Here's how the part is built. I have some questions about the finished solid (model axes, mm). Face numbers are marked on the shaded views. A direction names the side the tool comes from. Round coordinates to 2 decimals unless told otherwise and drop trailing zeros. Write each loop counter-clockwise with the first axis right and the second up, starting at its lowest first coordinate (ties: lowest second). Pieces come first, ordered by that corner, then holes. Notation, with made-up numbers: M 2.25,-23 L 17.25,-23 A9 ccw 17.25,-16 Z; hole C 28,72 d8. An arc over 180 degrees is marked long. Use a Markdown table: item, result. Add a question column.
Autodesk Inventor part; units mm, degrees
ref_plane "YZ Plane" through (0, 0, 0) normal (1, 0, 0) x (0, 1, 0)
ref_plane "XZ Plane" through (0, 0, 0) normal (0, 1, 0) x (-1, 0, 0)
ref_plane "XY Plane" through (0, 0, 0) normal (0, 0, 1) x (1, 0, 0)
sketch "Boceto1" plane through (0, 0, 0) normal (0, 1, 0) x (-1, 0, 0)
  line L0 (0, 0) -> (-200, 0)
  line L1 (-200, 0) -> (-200, -140)
  line L2 (-200, -140) -> (0, -140)
  line L3 (0, -140) -> (0, 0)
  line L4 (0, 0) -> (-200, 0)
  line L5 (-200, 0) -> (-200, -10)
  line L6 (-200, -10) -> (0, -10)
  line L7 (0, -10) -> (0, 0)
  line L8 (0, -140) -> (-200, -140)
  line L9 (-200, -140) -> (-200, -130)
  line L10 (-200, -130) -> (0, -130)
  line L11 (0, -130) -> (0, -140)
  dimension "d0" = 200
  dimension "d1" = 140
  dimension "d2" = 200
  dimension "d3" = 10
  dimension "d4" = 200
  dimension "d5" = 10
extrude "Extrusión1" add sketch "Boceto1" along normal blind 10 contours L3 L10 L1 L6
extrude "Extrusión2" add sketch "Boceto1" along normal blind 70 contours L3 L6 L1 L0 | L3 L2 L1 L10
properties part number "Soporte_rods" material "Acero, fundido"
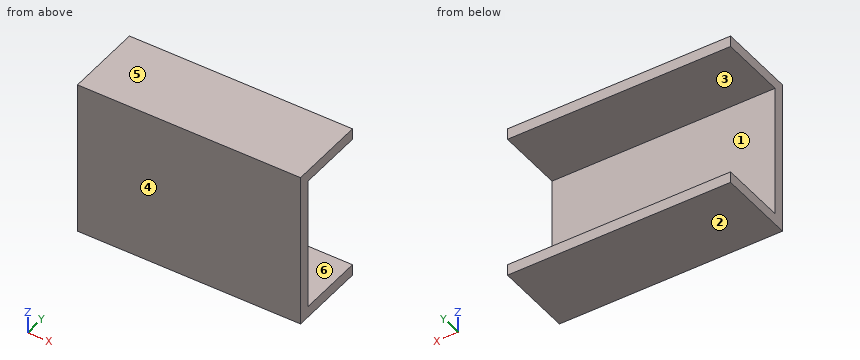
Item 1: I need wall thicknesses on probe 1 along Z at (x, y) = (41, 59); probe 2 along Y at (x, z) = (158, -20.5). Which ranges of each line are inside material? Lowest first, please. Write a range as from..to.
Item 2: Imagine slicing it at C-C on z = -87. List the corners of the cut face in (x, y) for me.
Item 3: On a 3-axis mill with a long thin cutter (end or side, diameter ignored), from which of +Z, -Z, +X, -X, +Y, -Y can I reach the whole of each face in a straight line? I mean the marked faces 1 and 2. Say none if no direction works.
Item 4: Imagine slicing it at B-B on y = 41. List the corners of the cut face in (x, z) for me, plus the area to 3 significant figures.
Item 5: If we mould it in two halves opening along Z, with no side actions, what happens to the marked faces 3, 4, 5 and 6? For each: +Z half, -Z half, draft (parallel to the pull), parting line (faces both ways), or undercut.
Item 6: Imagine slicing it at A-A on x = 21. List the corners of the cut face in (y, z) for me.
Item 7: For pin 1 Ø4 at (x, z) = (120, -60.5) entering from +Y, with a flat end and sliding along its axis, tell me the tip position at first contact or that it passes through.
The answers:
| question | item | result |
|---|---|---|
| 1 | probe 1 | -140..-130, -10..0 |
| 1 | probe 2 | 0..10 |
| 2 | outline | M 0,0 L 200,0 L 200,10 L 0,10 Z |
| 3 | face 1 | +X, -X, +Y |
| 3 | face 2 | -Z, +X, -X, +Y, -Y |
| 4 | outline | M 0,-140 L 200,-140 L 200,-130 L 0,-130 Z; M 0,-10 L 200,-10 L 200,0 L 0,0 Z |
| 4 | area | 4,000 mm² |
| 5 | face 3 | undercut |
| 5 | face 4 | draft |
| 5 | face 5 | +Z half |
| 5 | face 6 | undercut |
| 6 | outline | M 0,-140 L 70,-140 L 70,-130 L 10,-130 L 10,-10 L 70,-10 L 70,0 L 0,0 Z |
| 7 | pin 1 | y = 10 |
